from build123d import *

# Parameters (mm, degrees)
SALIENTE_EXTRUIR2_DEPTH = 6
REDONDEO1_R             = 0.1
CROQUIS3_W              = 2
CROQUIS3_H              = 3.3
CORTAR_EXTRUIR2_DEPTH   = 5
CROQUIS4_R              = 0.1
CORTAR_EXTRUIR3_DEPTH   = 6
CROQUIS5_W              = 0.5
CROQUIS5_H              = 3
CORTAR_EXTRUIR4_DEPTH   = 0.1


with BuildPart() as part:
    # Croquis1 → Saliente-Extruir2 (new body)
    with BuildSketch(Plane(origin=(0, 0, 0), x_dir=(1, 0, 0), z_dir=(0, 1, 0))):
        with BuildLine():
            Line((2.986733927, 4.5), (-10, 4.5))
            Line((-10, 4.5), (-10, -5))
            Line((-10, -5), (10, -5))
            Line((10, -5), (10, 5))
            Line((10, 5), (3.286733927, 5))
            Line((3.286733927, 5), (3.286733927, 4.8))
            ThreePointArc((3.286733927, 4.8), (3.198865961, 4.587867966), (2.986733927, 4.5))
        make_face()
    extrude(amount=SALIENTE_EXTRUIR2_DEPTH)

    # Redondeo1
    redondeo1_edges = [part.edges().sort_by_distance(p)[0] for p in [
        (3.286733927, 3, -5),
    ]]
    fillet(redondeo1_edges, radius=REDONDEO1_R)

    # Croquis3 → Cortar-Extruir2 (cut)
    with BuildSketch(Plane(origin=(0, 0, -4.5), x_dir=(-1, 0, 0), z_dir=(0, 0, -1))):
        with Locations((-0.386733927, 3)):
            Rectangle(CROQUIS3_W, CROQUIS3_H)
    extrude(amount=-CORTAR_EXTRUIR2_DEPTH, mode=Mode.SUBTRACT)

    # Croquis4 → Cortar-Extruir3 (cut)
    with BuildSketch(Plane(origin=(0, 6, 0), x_dir=(1, 0, 0), z_dir=(0, 1, 0))):
        with Locations(Location((6.3, 4, 0), (0, 0, 270))):
            Circle(CROQUIS4_R)
    extrude(amount=-CORTAR_EXTRUIR3_DEPTH, mode=Mode.SUBTRACT)

    # Croquis5 → Cortar-Extruir4 (cut)
    with BuildSketch(Plane.XY.offset(5)):
        with Locations((-8.247200411, 3)):
            Rectangle(CROQUIS5_W, CROQUIS5_H)
        with Locations((-0.947200411, 3)):
            Rectangle(CROQUIS5_W, CROQUIS5_H)
        with Locations((8.052799589, 3)):
            Rectangle(CROQUIS5_W, CROQUIS5_H)
    extrude(amount=-CORTAR_EXTRUIR4_DEPTH, mode=Mode.SUBTRACT)


solid = part.part
Geometry: final body of the model. Coordinates: model frame, mm. A direction names the side the tool comes from. Give positions to 0.01 mm unless a question says otherwise; leave off trailing zeros. Loops run counter-clockwise (first coordinate to the right, second up) from the corner with the lowest first, then second, coordinate; pieces in that order, holes last. Notation, with made-up numbers: (46.25, -11) - (91.25, -11) arc R18 cw to (91.25, 21) - close; hole circle Ø1 at (-33, 26.5). An arc over 180 degrees is marked (long way). Answer as CSV lines item,"result". Start each with the question number.
1. Section A-A, the plane z = -2. Return loops of the section in (x, y).
2. Section D-D, the plane y = 4.9. Return loops of the section in (x, z), plus the area to 3 significant figures.
3. Ray query, L1, parallel to X at y = 4.35, z = -4; L2, parallel to X at y = 3.1, z = -2.75; L3, parallel to Z at x = 6.3, y = 2.85. Return the intervals inside material, ascending.
4. Reachability of faces 1 (the face through (-3, 3, -4.5)), 2 (the face through (0, 1.35, -2)), 3 (the face through (7, 3, -5)) from +Z, -Z, +X, -X, +Y, -Y: full face, straight path, thin tool, end or side. Return the list, or none.
5. Draft query along Y for faces 4 (the face through (0, 3, 0.5)), 5 (the face through (0, 0, 0)), 6 (the face through (10, 3, 0)). Return one class per face: released by +Y, released by -Y, zero draft, split by the parting line, or undercut.
6. Section C-C, the plane x = -5. Return loops of the section in (y, z).
7. Pin query (flat end, axial travel): P1, Ø2, axis at x = -5.5, z = 2.5, coming from the -Y side; P2, Ø2, axis at x = 1, y = 3, coming from the -Z side. Return the tip coordinate at first contact, or that it passes through.
8. Section B-B, the plane y = 3.4. Return loops of the section in (x, z), plus the area to 3 significant figures.
Answers:
1,outline,"(-10, 0) - (10, 0) - (10, 6) - (-10, 6) - close; hole (-0.61, 1.35) - (1.39, 1.35) - (1.39, 4.65) - (-0.61, 4.65) - close"
2,outline,"(-10, -4.5) - (2.99, -4.5) arc R0.3 cw to (3.29, -4.8) - (3.29, -4.9) arc R0.1 ccw to (3.39, -5) - (10, -5) - (10, 5) - (-10, 5) - close; hole circle Ø0.2 at (6.3, -4)"
2,area,"193 mm2"
3,L1,"x = -10 to -0.61, 1.39 to 6.2, 6.4 to 10"
3,L2,"x = -10 to -0.61, 1.39 to 10"
3,L3,"z = -5 to -4.1, -3.9 to 5"
4,face 1,"-Z, -X, +Y, -Y"
4,face 2,"-Z"
4,face 3,"-Z, +X, -X, +Y, -Y"
5,face 4,"undercut"
5,face 5,"released by -Y"
5,face 6,"zero draft"
6,outline,"(0, -4.5) - (6, -4.5) - (6, 5) - (0, 5) - close"
7,P1,"stops at y = 0"
7,P2,"stops at z = -4.5"
8,outline,"(-10, -4.5) - (-0.61, -4.5) - (-0.61, 0.5) - (1.39, 0.5) - (1.39, -4.5) - (2.99, -4.5) arc R0.3 cw to (3.29, -4.8) - (3.29, -4.9) arc R0.1 ccw to (3.39, -5) - (10, -5) - (10, 5) - (8.3, 5) - (8.3, 4.9) - (7.8, 4.9) - (7.8, 5) - (-0.7, 5) - (-0.7, 4.9) - (-1.2, 4.9) - (-1.2, 5) - (-8, 5) - (-8, 4.9) - (-8.5, 4.9) - (-8.5, 5) - (-10, 5) - close; hole circle Ø0.2 at (6.3, -4)"
8,area,"183 mm2"
